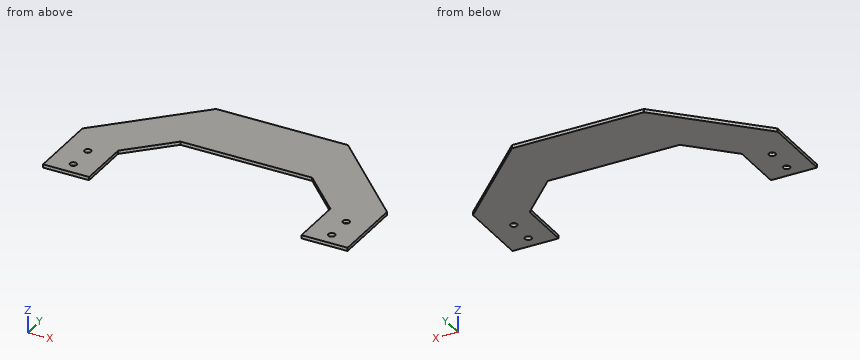
```python
from build123d import *

# Parameters (mm, degrees)
BOSS_EXTRUDE1_DEPTH = 3.175
SKETCH4_R           = 3.175
CUT_EXTRUDE2_DEPTH  = 3.175


with BuildPart() as part:
    # Sketch1 → Boss-Extrude1 (new body)
    with BuildSketch(Plane.XY):
        Polygon((-63.5, 31.430896424), (-146.688207153, -51.757310729), (-146.688207153, -120.969103576), (-102.238207153, -120.969103576), (-102.238207153, -70.169103576), (-63.5, -31.430896424), (0, -31.430896424), (0, 31.430896424), align=None)
    boss_extrude1 = extrude(amount=BOSS_EXTRUDE1_DEPTH)

    # Sketch4 → Cut-Extrude2 (cut)
    with BuildSketch(Plane.XY.offset(3.175)):
        with Locations((-124.463207153, -108.269103576)):
            Circle(SKETCH4_R)
        with Locations((-124.463207153, -82.869103576)):
            Circle(SKETCH4_R)
    cut_extrude2 = extrude(amount=-CUT_EXTRUDE2_DEPTH, mode=Mode.SUBTRACT)

    # Mirror4: Boss-Extrude1, Cut-Extrude2 across plane
    add(boss_extrude1.mirror(Plane(origin=(0, 31.430896424, 3.175), x_dir=(0, 0, 1), z_dir=(-1, 0, 0))))
    add(cut_extrude2.mirror(Plane(origin=(0, 31.430896424, 3.175), x_dir=(0, 0, 1), z_dir=(-1, 0, 0))), mode=Mode.SUBTRACT)


solid = part.part
```
Model file for the job. Use its own axes, mm. Give positions to 0.01 mm unless a question says otherwise; leave off trailing zeros. Write each loop counter-clockwise with the first axis right and the second up, starting at its lowest first coordinate (ties: lowest second). Pieces come first, ordered by that corner, then holes. Notation, with made-up numbers: (79.5, 85.5) -> (89.5, 85.5) arc R10 ccw to (89.5, 102.5) -> close; hole circle Ø5 at (56.25, -35). An arc over 180 degrees is marked (long way). Use CSV: the item, a comma, the result in double quotes. Start each with the question number.
1) Cut at D-D on y = -22.5. List the corners of the cut face in (x, z) (3 decimals).
2) Cut at C-C on x = 48.5. List the corners of the cut face in (y, z) (3 decimals).
3) Pin check, flat tip, straight feed: P1, Ø1.5, axis at y = -40, z = 0.5, coming from the +X side. Stop position of the tip, or through.
4) Cut at A-A on y = -66. List the corners of the cut face in (x, z) (3 decimals), plus the area to 3 significant figures.
5) Drill centre lines: L1, parallel to X at y = -89.5, z = 1.55; L2, parallel to Y at x = 14.5, z = 2.35; L3, parallel to X at y = -69, z = 2.35. Where is each one in solid material? Low to high.
6) Cut at B-B on z = 1.5. List the corners of the cut face in (x, y) (3 decimals), plus the area to 3 significant figures.
Final values:
1,outline,"(-117.431, 0) -> (117.431, 0) -> (117.431, 3.175) -> (-117.431, 3.175) -> close"
2,outline,"(-31.431, 0) -> (31.431, 0) -> (31.431, 3.175) -> (-31.431, 3.175) -> close"
3,P1,"stops at x = 135.68"
4,outline,"(-146.688, 0) -> (-98.069, 0) -> (-98.069, 3.175) -> (-146.688, 3.175) -> close; (98.069, 0) -> (146.688, 0) -> (146.688, 3.175) -> (98.069, 3.175) -> close"
4,area,"309 mm2"
5,L1,"x = -146.69 to -102.24, 102.24 to 146.69"
5,L2,"y = -31.43 to 31.43"
5,L3,"x = -146.69 to -101.07, 101.07 to 146.69"
6,outline,"(-146.688, -120.969) -> (-102.238, -120.969) -> (-102.238, -70.169) -> (-63.5, -31.431) -> (63.5, -31.431) -> (102.238, -70.169) -> (102.238, -120.969) -> (146.688, -120.969) -> (146.688, -51.757) -> (63.5, 31.431) -> (-63.5, 31.431) -> (-146.688, -51.757) -> close; hole circle Ø6.35 at (-124.463, -108.269); hole circle Ø6.35 at (-124.463, -82.869); hole circle Ø6.35 at (124.463, -108.269); hole circle Ø6.35 at (124.463, -82.869)"
6,area,"20,900 mm2"
